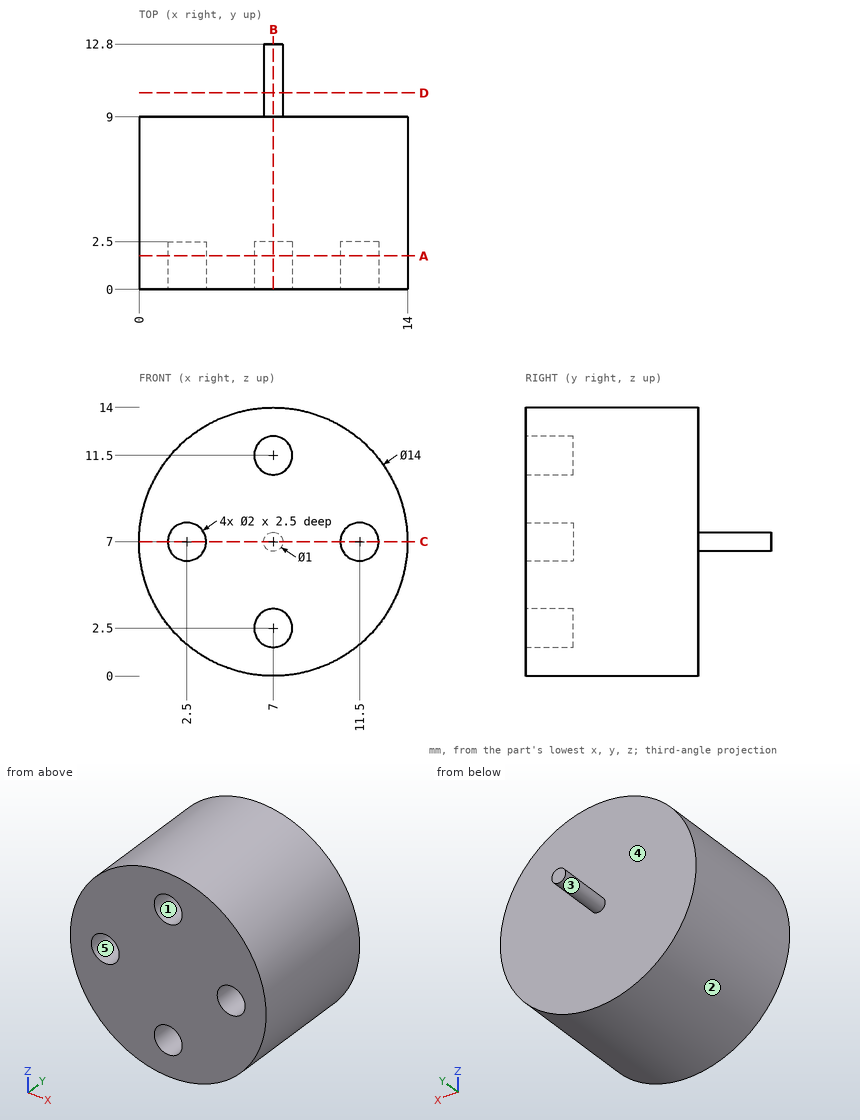
Input: dimensioned drawing with shaded views. Units: mm. Origin: part minimum x, y, z. A direction names the side the tool comes from. Coordinates: 2 decimals unless noted, no trailing zeros. Order: outer loops, then holes, each group sorted by start corner. A loop starts at its lowest first (then second) coordinate and runs counter-clockwise, first axis right, second up.
Item 1: Access query for the marked faces 1 and 2. Directions: +Z, -Z, +X, -X, +Y, -Y. A direction counts if a zero-diameter tool reaches every point of the face in a straight line with its end or side. Return the directions, or none.
Answer:
face 1: -Y
face 2: +Y, -Y
Item 2: Section query A-A (y = 1.75). Output: boundary loops of the cut face in (x, z).
Answer:
outline: circle Ø14 at (7, 7); hole circle Ø2 at (2.5, 7); hole circle Ø2 at (7, 2.5); hole circle Ø2 at (7, 11.5); hole circle Ø2 at (11.5, 7)
Item 3: Draft query along Z for the marked faces 3, 4 and 5. Return one class per face: released by +Z, released by -Z, zero draft, split by the parting line, or undercut.
Answer:
face 3: split by the parting line
face 4: zero draft
face 5: undercut
Item 4: Section query D-D (y = 10.25). Output: boundary loops of the cut face in (x, z), then the cut area to 3 significant figures.
Answer:
outline: circle Ø1 at (7, 7)
area: 0.785 mm2
Item 5: Section query B-B (x = 7). Output: boundary loops of the cut face in (y, z), then the cut area to 3 significant figures.
Answer:
outline: (0, 0) - (9, 0) - (9, 6.5) - (12.8, 6.5) - (12.8, 7.5) - (9, 7.5) - (9, 14) - (0, 14) - (0, 12.5) - (2.5, 12.5) - (2.5, 10.5) - (0, 10.5) - (0, 3.5) - (2.5, 3.5) - (2.5, 1.5) - (0, 1.5) - close
area: 120 mm2
Item 6: Section query C-C (z = 7). Output: boundary loops of the cut face in (x, y).
Answer:
outline: (0, 0) - (1.5, 0) - (1.5, 2.5) - (3.5, 2.5) - (3.5, 0) - (10.5, 0) - (10.5, 2.5) - (12.5, 2.5) - (12.5, 0) - (14, 0) - (14, 9) - (7.5, 9) - (7.5, 12.8) - (6.5, 12.8) - (6.5, 9) - (0, 9) - close
Item 7: Contact query for flat-ended pins moving along their axis: P1, Ø5, axis at x = 11.5, z = 6, coming from the -Y side; P2, Ø1.6, axis at x = 7, z = 11.5, coming from the +Y side; P3, Ø1.6, axis at x = 2.5, z = 7, coming from the -Y side; P4, Ø5, axis at y = 10.5, z = 11, coming from the +X side. Output: stop coordinate, or through.
Answer:
P1: stops at y = 0
P2: stops at y = 9
P3: stops at y = 2.5
P4: stops at x = 13.71
Item 8: Material intervals for line 1 along X through (y, z) = (1.9, 7); line 2 along Y through (x, z) = (6.75, 13.25); line 3 along X through (y, z) = (1.5, 2.5), sorted ascending.
Answer:
line 1: x = 0 to 1.5, 3.5 to 10.5, 12.5 to 14
line 2: y = 0 to 9
line 3: x = 1.64 to 6, 8 to 12.36
